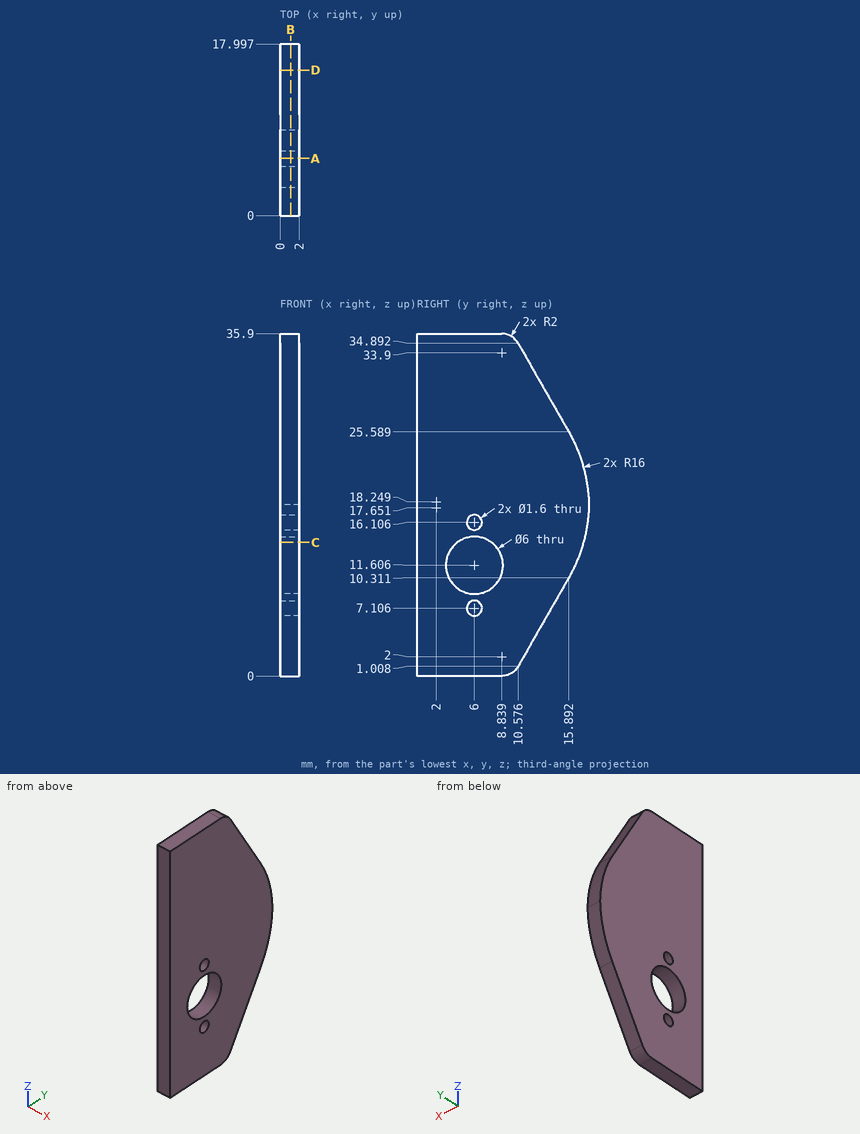
Job drawing, mm, ordinate dimensions from the low corner. One solid piece. Give positions to 0.01 mm unless a question says otherwise; leave off trailing zeros. Order: outer loops, then holes, each group sorted by start corner. A loop starts at its lowest first (then second) coordinate and runs counter-clockwise, first axis right, second up. Notation, with made-up numbers: (71.5, 22) - (112.5, 22) arc R15 ccw to (112.5, 49) - close; hole circle Ø7 at (70.25, -34.5). An arc over 180 degrees is marked (long way). Return JSON: item names as keys, results as strings.
1) Flat gauge pin, fed straight in: P1, Ø1.3, axis at y = 6, z = 7.11, coming from the -X side. Where does the tip first touch, or does it go through?
Geometry says:
{"P1": "through"}
2) Cut at A-A, the plane y = 6. Give the cut face in (x, z) (1 decimal).
Geometry says:
{"outline": "(0, 0) - (2, 0) - (2, 6.3) - (0, 6.3) - close; (0, 7.9) - (2, 7.9) - (2, 8.6) - (0, 8.6) - close; (0, 14.6) - (2, 14.6) - (2, 15.3) - (0, 15.3) - close; (0, 16.9) - (2, 16.9) - (2, 35.9) - (0, 35.9) - close"}
3) Cut at C-C, the plane z = 14. Give the cut face in (x, y) (1 decimal), plus the area to 3 significant figures.
Geometry says:
{"outline": "(0, 0) - (2, 0) - (2, 4.2) - (0, 4.2) - close; (0, 7.8) - (2, 7.8) - (2, 17.4) - (0, 17.4) - close", "area": "27.6 mm²"}
4) Cut at B-B, the plane x = 1.1. Count the separate pieces of the cut face and the enclosed holes in it, plus the area to 3 significant figures.
Geometry says:
{"separate pieces": "1", "enclosed holes": "3", "area": "498 mm²"}
5) Cut at D-D, the plane y = 15.25. Give the cut face in (x, z).
Geometry says:
{"outline": "(0, 9.19) - (2, 9.19) - (2, 26.71) - (0, 26.71) - close"}
6) Probe line 1 (Y direction, x = 0.5, z = 10) (1 decimal); line 2 (Y direction, x = 0.25, z = 13.5) (1 decimal); line 3 (Z direction, x = 1.2, y = 8). List the from-to ranges inside material, lowest first. Write a range as from..to.
Geometry says:
{"line 1": "0..3.5, 8.5..15.7", "line 2": "0..3.7, 8.3..17.3", "line 3": "0..9.37, 13.84..35.9"}
